Verification items for the finished model (mm, model axes). Face numbers are marked on the shaded views. A direction names the side the tool comes from. Give positions to 0.01 mm unless a question says otherwise; leave off trailing zeros. Loops run counter-clockwise (first coordinate to the right, second up) from the corner with the lowest first, then second, coordinate; pieces in that order, holes last. Notation, with made-up numbers: M 46.25,57 L 103.25,57 A6 ccw 103.25,62 Z; hole C 79,3.5 d5. An arc over 180 degrees is marked long. Use CSV: the item, a comma, the result in double quotes.
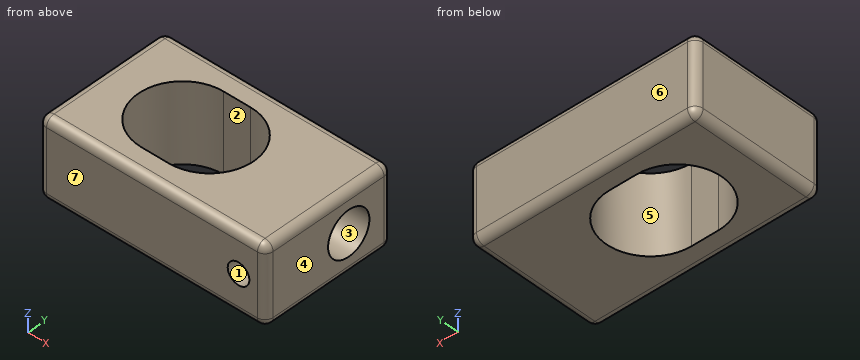
from build123d import *

# Parameters (mm, degrees)
BOSS_EXTRUDE1_DEPTH      = 7.25
BOSS_EXTRUDE1_DEPTH_BACK = 7.25
SKETCH1_W                = 42
SKETCH1_H                = 25
SKETCH2_R                = 4.1
CUT_EXTRUDE1_DEPTH       = 12
SKETCH3_R                = 2
CUT_EXTRUDE5_DEPTH       = 15
FILLET3_R                = 1.5


with BuildPart() as part:
    # Sketch1 → Boss-Extrude1 (new, two sides: drawn at the far end of the back side and taken through both)
    with BuildSketch(Plane.XY.offset(-BOSS_EXTRUDE1_DEPTH_BACK)):
        with Locations((-44, 0)):
            Rectangle(SKETCH1_W, SKETCH1_H)
        with BuildLine():
            Line((-45, -8.15), (-50, -8.15))
            ThreePointArc((-50, -8.15), (-58.15, 0), (-50, 8.15))
            Line((-50, 8.15), (-45, 8.15))
            ThreePointArc((-45, 8.15), (-36.85, 0), (-45, -8.15))
        make_face(mode=Mode.SUBTRACT)
    extrude(amount=BOSS_EXTRUDE1_DEPTH + BOSS_EXTRUDE1_DEPTH_BACK)

    # Sketch2 → Cut-Extrude1 (cut)
    with BuildSketch(Plane(origin=(-23, 0, 0), x_dir=(0, 0, -1), z_dir=(1, 0, 0))):
        with Locations(Location((0, 4, 0), (0, 0, 90))):
            Circle(SKETCH2_R)
    extrude(amount=-CUT_EXTRUDE1_DEPTH, mode=Mode.SUBTRACT)

    # Sketch3 → Cut-Extrude5 (cut)
    with BuildSketch(Plane(origin=(0, -12.5, 0), x_dir=(1, 0, 0), z_dir=(0, 1, 0))):
        with Locations(Location((-28, 0, 0), (0, 0, 90))):
            Circle(SKETCH3_R)
    extrude(amount=CUT_EXTRUDE5_DEPTH, mode=Mode.SUBTRACT)

    # Fillet3
    fillet3_edges = [part.edges().sort_by_distance(p)[0] for p in [
        (-23, 0, -7.25),
        (-44, 12.5, -7.25),
        (-65, 0, 7.25),
        (-44, -12.5, 7.25),
        (-23, 0, 7.25),
        (-44, 12.5, 7.25),
        (-65, 0, -7.25),
        (-65, 12.5, 0),
        (-23, 12.5, 0),
        (-23, -12.5, 0),
        (-65, -12.5, 0),
        (-44, -12.5, -7.25),
    ]]
    fillet(fillet3_edges, radius=FILLET3_R)


solid = part.part
(1) Section check B-B on x = -46.5. Record the cut outline in (y, z).
Calculated:
outline,"M -12.5,-5.75 A1.5 ccw -11,-7.25 L -8.15,-7.25 L -8.15,7.25 L -11,7.25 A1.5 ccw -12.5,5.75 Z; M 8.15,-7.25 L 11,-7.25 A1.5 ccw 12.5,-5.75 L 12.5,5.75 A1.5 ccw 11,7.25 L 8.15,7.25 Z"
(2) Depth check by flat-ended pin: pin 1 Ø2.5 at (x, z) = (-28, 0) entering from -Y. Enter the tip coordinate at first touch or a pass-through.
Calculated:
pin 1,"stops at y = 7.9"
(3) Section check A-A on z = 0. Record the cut outline in (x, y).
Calculated:
outline,"M -65,-11 A1.5 ccw -63.5,-12.5 L -30,-12.5 L -30,-0.1 L -35,-0.1 L -35,8.1 L -23,8.1 L -23,11 A1.5 ccw -24.5,12.5 L -63.5,12.5 A1.5 ccw -65,11 Z; M -26,-12.5 L -24.5,-12.5 A1.5 ccw -23,-11 L -23,-0.1 L -26,-0.1 Z; hole M -50,-8.15 L -45,-8.15 A8.15 ccw -45,8.15 L -50,8.15 A8.15 ccw Z"
(4) Tool access check on the marked faces 1, 2 and 3. Record the directions out of +Z, -Z, +X, -X, +Y, -Y that give a thin tool (end or side, any length) a straight path to the whole face; none if there is none.
Calculated:
face 1,"-Y"
face 2,"+Z, -Z"
face 3,"+X"
(5) Section check C-C on z = -5.25. Record the cut outline in (x, y).
Calculated:
outline,"M -65,-11 A1.5 ccw -63.5,-12.5 L -24.5,-12.5 A1.5 ccw -23,-11 L -23,11 A1.5 ccw -24.5,12.5 L -63.5,12.5 A1.5 ccw -65,11 Z; hole M -50,-8.15 L -45,-8.15 A8.15 ccw -45,8.15 L -50,8.15 A8.15 ccw Z"
(6) Scan lines: L1, parallel to Y at x = -46.5, z = -5.5; L2, parallel to Y at x = -31, z = 0; L3, parallel to X at y = -2.25, z = 0. Record each from-to range of solid material in increasing order. Write a range as from..to.
Calculated:
L1,"y = -12.5..-8.15, 8.15..12.5"
L2,"y = -12.5..-0.1, 8.1..12.5"
L3,"x = -65..-57.83, -37.17..-30, -26..-23"
(7) Section check D-D on x = -33. Record the cut outline in (y, z), plus the area to 3 significant figures.
Calculated:
outline,"M -12.5,-5.75 A1.5 ccw -11,-7.25 L 11,-7.25 A1.5 ccw 12.5,-5.75 L 12.5,5.75 A1.5 ccw 11,7.25 L -11,7.25 A1.5 ccw -12.5,5.75 Z; hole C 4,0 d8.2"
area,"308 mm²"
(8) Mould release check, pull along Y, two halves, no side actions. Record for the marked faces 4, 5, 6 and 7: released by +Y, released by -Y, zero draft, split by the parting line, or undercut.
Calculated:
face 4,"zero draft"
face 5,"undercut"
face 6,"released by +Y"
face 7,"released by -Y"
